from build123d import *

# Parameters (mm, degrees)
SKETCH1_R           = 3.175
BOSS_EXTRUDE2_DEPTH = 4.0005
FILLET1_R           = 6.35
SKETCH6_R           = 1.7
CUT_EXTRUDE2_DEPTH  = 253.287066958
SKETCH5_W           = 42
SKETCH5_H           = 22
CUT_EXTRUDE1_DEPTH  = 253.287066958


with BuildPart() as part:
    # Sketch1 → Boss-Extrude2 (new, symmetric)
    with BuildSketch(Plane.YZ):
        Polygon((-41.275, 114.3), (-41.275, -114.3), (41.275, -114.3), (41.275, 114.3), (0, 266.7), align=None)
        with Locations(Location((0, 0, 0), (0, 0, 270))):
            Circle(SKETCH1_R, mode=Mode.SUBTRACT)
    extrude(amount=BOSS_EXTRUDE2_DEPTH, both=True)

    # Fillet1
    fillet1_edges = [part.edges().sort_by_distance(p)[0] for p in [
        (0, 0, 266.7),
        (0, 41.275, 114.3),
        (0, 41.275, -114.3),
        (0, -41.275, -114.3),
        (0, -41.275, 114.3),
    ]]
    fillet(fillet1_edges, radius=FILLET1_R)

    # Sketch6 → Cut-Extrude2 (cut, through all)
    with BuildSketch(Plane.YZ.offset(4.0005)):
        with Locations(Location((-34.75, -92.95, 0), (0, 0, 270))):
            Circle(SKETCH6_R)
        with Locations(Location((-34.75, -102.95, 0), (0, 0, 270))):
            Circle(SKETCH6_R)
        with Locations(Location((14.75, -92.95, 0), (0, 0, 270))):
            Circle(SKETCH6_R)
        with Locations(Location((14.75, -102.95, 0), (0, 0, 270))):
            Circle(SKETCH6_R)
    extrude(amount=-CUT_EXTRUDE2_DEPTH, mode=Mode.SUBTRACT)

    # Sketch5 → Cut-Extrude1 (cut, through all)
    with BuildSketch(Plane.YZ.offset(4.0005)):
        with Locations((-10, -97.95)):
            Rectangle(SKETCH5_W, SKETCH5_H)
    extrude(amount=-CUT_EXTRUDE1_DEPTH, mode=Mode.SUBTRACT)


solid = part.part
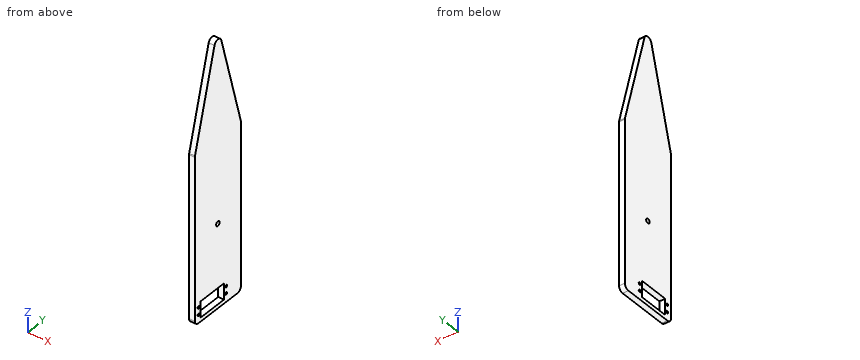
Check sheet for the modelled part. Datum: model origin and axes. Units: mm. Give positions to 0.01 mm unless a question says otherwise; leave off trailing zeros. Write each loop counter-clockwise with the first axis right and the second up, starting at its lowest first coordinate (ties: lowest second). Pieces come first, ordered by that corner, then holes. Notation, with made-up numbers: (-9, 89.25) -> (-4, 89.25) arc R18 cw to (-4, 106.25) -> close; hole circle Ø5 at (59.25, 52). An arc over 180 degrees is marked (long way). Use one line per item in the form item = value. Start each with the question number.
1. Section check B-B (z = 0). Record the cut outline in (x, y) (1 decimal).
2. Go/stop test with flat-tipped pins: P1, Ø3, axis at y = 14.75, z = -102.95, coming from the -X side; P2, Ø1.5, axis at x = -0.5, z = 212.5, coming from the -Y side; P3, Ø5.5, axis at y = -34.75, z = -102.95, coming from the -X side. Record where each tip stops, or that it passes through.
3. Section check D-D (y = -20.5). Record the cut outline in (x, z), and give its area (3 significant figures).
4. Thickness scan on line 1 along Y through (x, z) = (-0.25, -102.95) (3 decimals); line 2 along Z through (x, y) = (2, -1.5); line 3 along Y through (x, z) = (-1, 0) (3 decimals). Record the ranges inside material, lowest first. Write a range as from..to.
5. Section check C-C (x = 0.5). Record the cut outline in (y, z) (3 decimals).
6. Section check A-A (y = 0). Count the separate pieces of the cut face and the enclosed holes in it, and give its area (3 significant figures).
Conclusion:
q1.outline = (-4, -41.3) -> (4, -41.3) -> (4, -3.2) -> (-4, -3.2) -> close; (-4, 3.2) -> (4, 3.2) -> (4, 41.3) -> (-4, 41.3) -> close
q2.P1 = through
q2.P2 = -14.88
q2.P3 = -4
q3.outline = (-4, -114.3) -> (4, -114.3) -> (4, -108.95) -> (-4, -108.95) -> close; (-4, -86.95) -> (4, -86.95) -> (4, 191.01) -> (-4, 191.01) -> close
q3.area = 2,270 mm²
q4.line_1 = -41.275..-36.45, -33.05..-31, 11..13.05, 16.45..41.275
q4.line_2 = -114.3..-108.95, -86.95..-2.8, 2.8..248.58
q4.line_3 = -41.275..-3.175, 3.175..41.275
q5.outline = (-41.275, -107.95) arc R6.35 ccw to (-34.925, -114.3) -> (34.925, -114.3) arc R6.35 ccw to (41.275, -107.95) -> (41.275, 113.455) arc R6.35 ccw to (41.054, 115.115) -> (6.129, 244.069) arc R6.35 ccw to (-6.129, 244.069) -> (-41.054, 115.115) arc R6.35 ccw to (-41.275, 113.455) -> close; hole circle Ø3.4 at (-34.75, -102.95); hole circle Ø3.4 at (-34.75, -92.95); hole (-31, -108.95) -> (11, -108.95) -> (11, -86.95) -> (-31, -86.95) -> close; hole circle Ø6.35 at (0, 0); hole circle Ø3.4 at (14.75, -102.95); hole circle Ø3.4 at (14.75, -92.95)
q6.separate_pieces = 3
q6.enclosed_holes = 0
q6.area = 2,680 mm²
